Check sheet for the modelled part. Datum: model origin and axes. Units: mm. Face numbers are marked on the shaded views. A direction names the side the tool comes from. Give positions to 0.01 mm unless a question says otherwise; leave off trailing zeros. Loops run counter-clockwise (first coordinate to the right, second up) from the corner with the lowest first, then second, coordinate; pieces in that order, holes last. Notation, with made-up numbers: M 70.25,23.5 L 119.25,23.5 A23 cw 119.25,55.5 Z; hole C -30.75,31 d9. An arc over 180 degrees is marked long. Use one line per item in the form item = value.
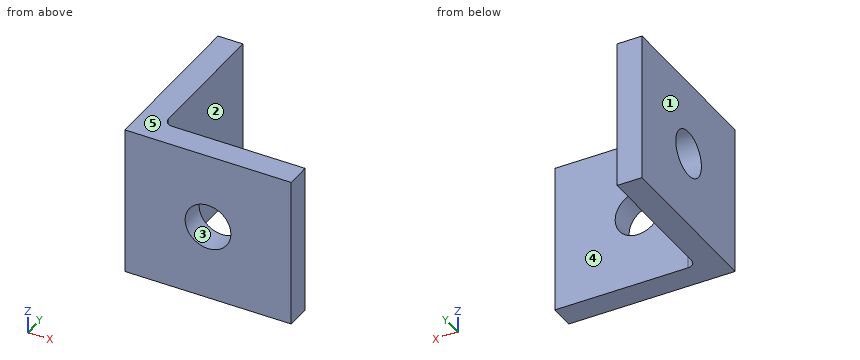
from build123d import *

# Parameters (mm, degrees)
BOSS_EXTRUDE1_DEPTH = 9
SKETCH2_R           = 2.75
CUT_EXTRUDE1_DEPTH  = 4
SKETCH3_R           = 2.75
CUT_EXTRUDE2_DEPTH  = 4


with BuildPart() as part:
    # Sketch1 → Boss-Extrude1 (new body, symmetric)
    with BuildSketch(Plane.XY):
        with BuildLine():
            Line((0, 0), (0, 20))
            Line((0, 20), (3, 20))
            Line((3, 20), (3, 4))
            ThreePointArc((3, 4), (3.292893219, 3.292893219), (4, 3))
            Line((4, 3), (20, 3))
            Line((20, 3), (20, 0))
            Line((20, 0), (0, 0))
        make_face()
    extrude(amount=BOSS_EXTRUDE1_DEPTH, both=True)

    # Sketch2 → Cut-Extrude1 (cut, through all)
    with BuildSketch(Plane(origin=(0, 3, 0), x_dir=(1, 0, 0), z_dir=(0, 1, 0))):
        with Locations((10, 0)):
            Circle(SKETCH2_R)
    extrude(amount=-CUT_EXTRUDE1_DEPTH, mode=Mode.SUBTRACT)

    # Sketch3 → Cut-Extrude2 (cut, through all)
    with BuildSketch(Plane(origin=(3, 0, 0), x_dir=(0, 0, -1), z_dir=(1, 0, 0))):
        with Locations((0, 10)):
            Circle(SKETCH3_R)
    extrude(amount=-CUT_EXTRUDE2_DEPTH, mode=Mode.SUBTRACT)


solid = part.part
1) Depth check by flat-ended pin: pin 1 Ø7 at (y, z) = (10, 0) entering from -X; pin 2 Ø8 at (y, z) = (10.5, 3.5) entering from +X. Enter the tip coordinate at first touch or a pass-through.
Evaluation:
pin_1 = 0
pin_2 = 3
2) Section check C-C (z = -4.5). Record the cut outline in (x, y).
Evaluation:
outline = M 0,0 L 20,0 L 20,3 L 4,3 A1 cw 3,4 L 3,20 L 0,20 Z
3) Scan lines: line 1 (Z direction, x = 10, y = 1.1); line 2 (X direction, y = 1.45, z = 0). Record each from-to range of solid material in increasing order.
Evaluation:
line_1 = -9 to -2.75, 2.75 to 9
line_2 = 0 to 7.25, 12.75 to 20
4) Release check for a two-part mould opening along Z. For the marked faces 3, 4 and 5 record: pulls with the +Z half, pulls with the -Z half, needs draft (parallel to the pull), parting line crosses it, or undercut.
Evaluation:
face_3 = undercut
face_4 = needs draft
face_5 = pulls with the +Z half
5) Set-up check for the marked faces 1 and 2: record each of +Z, -Z, +X, -X, +Y, -Y from which the full face is reachable in a straight line by a thin tool's end or side.
Evaluation:
face_1 = +Z, -Z, -X, +Y, -Y
face_2 = +Z, -Z, +X, +Y
6) Section check A-A (y = 10). Record the cut outline in (x, z).
Evaluation:
outline = M 0,-9 L 3,-9 L 3,-2.75 L 0,-2.75 Z; M 0,2.75 L 3,2.75 L 3,9 L 0,9 Z
7) Section check D-D (x = 16). Record the cut outline in (y, z), then the cut area to 3 significant figures.
Evaluation:
outline = M 0,-9 L 3,-9 L 3,9 L 0,9 Z
area = 54.0 mm^2
